from build123d import *

# Parameters (mm, degrees)
F0_W      = 250
F0_H      = 150
F1_DEPTH  = 30
F2_SIZE   = 3
F3_SIZE   = 3
F4_SIZE   = 3
F5_SIZE   = 3
F6_W      = 110
F6_H      = 60
F7_DEPTH  = 15
F8_SIZE   = 3
F9_R      = 7.216075
F9_R_2    = 5.170271
F9_R_3    = 7.754468
F9_R_4    = 5.863946
F9_R_5    = 7.338113
F9_R_6    = 5.427253
F9_R_7    = 7.074755
F9_R_8    = 4.927232
F10_DEPTH = 15


with BuildPart() as f1:
    # F0 (on Front) → F1 (new body)
    with BuildSketch(Plane.XZ):
        with Locations((10.972098, 17.180756)):
            Rectangle(F0_W, F0_H)
    extrude(amount=F1_DEPTH)

    # F2
    f2_edges = [f1.edges().sort_by_distance(p)[0] for p in [
        (-114.027902, -15, -57.819244),
    ]]
    chamfer(f2_edges, length=F2_SIZE)

    # F3
    f3_edges = [f1.edges().sort_by_distance(p)[0] for p in [
        (135.972098, -15, -57.819244),
    ]]
    chamfer(f3_edges, length=F3_SIZE)

    # F4
    f4_edges = [f1.edges().sort_by_distance(p)[0] for p in [
        (135.972098, -15, 92.180756),
    ]]
    chamfer(f4_edges, length=F4_SIZE)

    # F5
    f5_edges = [f1.edges().sort_by_distance(p)[0] for p in [
        (-114.027902, -15, 92.180756),
    ]]
    chamfer(f5_edges, length=F5_SIZE)

    # F6 (on face) → F7 (join)
    with BuildSketch(Plane.XZ.offset(30)):
        with Locations((10.972098, 17.180756)):
            Rectangle(F6_W, F6_H)
    extrude(amount=F7_DEPTH)

    # F8
    f8_edges = [f1.edges().sort_by_distance(p)[0] for p in [
        (-44.027902, -37.5, -12.819244),
        (-44.027902, -37.5, 47.180756),
        (65.972098, -37.5, -12.819244),
        (65.972098, -37.5, 47.180756),
    ]]
    chamfer(f8_edges, length=F8_SIZE)

    # F9 (on face) → F10 (join)
    with BuildSketch(Plane.XZ.offset(30)):
        with Locations((-93.364298, -44.450238)):
            Circle(F9_R)
        with Locations((-93.364298, -44.450238)):
            Circle(F9_R_2, mode=Mode.SUBTRACT)
        with Locations((112.311885, -44.177815)):
            Circle(F9_R_3)
        with Locations((112.311885, -44.177815)):
            Circle(F9_R_4, mode=Mode.SUBTRACT)
        with Locations((112.856723, 78.683056)):
            Circle(F9_R_5)
        with Locations((112.856723, 78.683056)):
            Circle(F9_R_6, mode=Mode.SUBTRACT)
        with Locations((-94.998814, 78.683056)):
            Circle(F9_R_7)
        with Locations((-94.998814, 78.683056)):
            Circle(F9_R_8, mode=Mode.SUBTRACT)
    extrude(amount=F10_DEPTH)


solid = f1.part
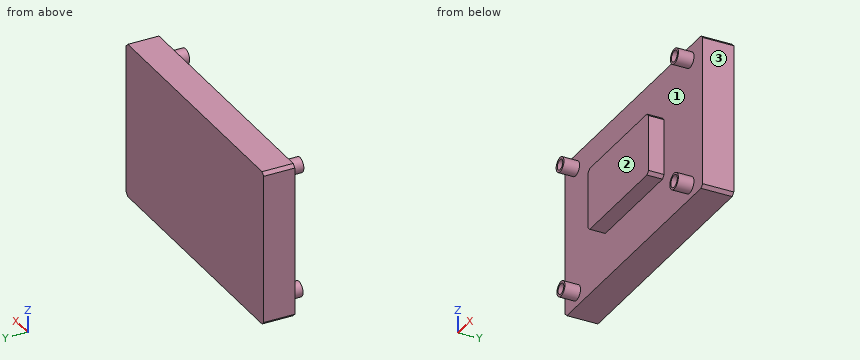
Design review of the part built by this model. Coordinates are the model's own, in mm. Face numbers are marked on the shaded views. Round coordinates to 2 decimals unless told otherwise and drop trailing zeros. Write each loop counter-clockwise with the first axis right and the second up, starting at its lowest first coordinate (ties: lowest second). Pieces come first, ordered by that corner, then holes. Notation, with made-up numbers: (37.25, -8.75) - (48.25, -8.75) arc R21 ccw to (48.25, -3.75) - close; hole circle Ø11 at (-23.75, -32). An arc over 180 degrees is marked (long way). Use a Markdown table: item, result. Add a question column.
1. We need section A-A (y = -37). Count the separate pieces of the cut face and the enclosed holes in it, then the cut area to 3 significant figures.
2. Wall thickness on probe 1 along Y at (x, z) = (-99, 41); probe 2 along X at (y, z) = (-30.5, 4.5): over which ranges is each line inside the solid? List them lowest first.
3. We need section C-C (x = 12). State the section outline as (y, z) points, then the cut area to 3 significant figures.
4. We need section B-B (z = 1). State the section outline as (x, y) points.
5. We need section D-D (z = 50). State the section outline as (x, y) points, then the cut area to 3 significant figures.
6. Clearance check with flat-ended pins moving along their axes: pin 1 (10 mm diameter, centred on x = 112.86, z = 78.68, fed in from -Y); pin 2 (12 mm diameter, centred on x = -6, y = -38.5, fed in from -Z); pin 3 (4.5 mm diameter, centred on x = 21.5, y = -39, fed in from +Z). State where each tip first meets the part, or that it passes through.
7. Mouldability with a two-part tool opening along X and no side actions: class the marked faces 1, 2 and 3 as +X half, -X half, draft (parallel to the pull), parting line (faces both ways), or undercut.
Output:
| question | item | result |
|---|---|---|
| 1 | separate pieces | 5 |
| 1 | enclosed holes | 4 |
| 1 | area | 6,900 mm2 |
| 2 | probe 1 | y = -30 to 0 |
| 2 | probe 2 | x = -44.03 to 65.97 |
| 3 | outline | (-45, -12.82) - (-30, -12.82) - (-30, -57.82) - (0, -57.82) - (0, 92.18) - (-30, 92.18) - (-30, 47.18) - (-45, 47.18) - close |
| 3 | area | 5,400 mm2 |
| 4 | outline | (-114.03, -30) - (-44.03, -30) - (-44.03, -45) - (65.97, -45) - (65.97, -30) - (135.97, -30) - (135.97, 0) - (-114.03, 0) - close |
| 5 | outline | (-114.03, -30) - (135.97, -30) - (135.97, 0) - (-114.03, 0) - close |
| 5 | area | 7,500 mm2 |
| 6 | pin 1 | stops at y = -30 |
| 6 | pin 2 | stops at z = -12.82 |
| 6 | pin 3 | stops at z = 47.18 |
| 7 | face 1 | undercut |
| 7 | face 2 | draft |
| 7 | face 3 | +X half |
